Geometry check sheet. Reference: the model listing, model coordinates, mm. A direction names the side the tool comes from. Round coordinates to 2 decimals unless told otherwise and drop trailing zeros. Write each loop counter-clockwise with the first axis right and the second up, starting at its lowest first coordinate (ties: lowest second). Pieces come first, ordered by that corner, then holes. Notation, with made-up numbers: (50.5, 39.5) - (75.5, 39.5) arc R13 ccw to (75.5, 62.5) - close; hole circle Ø10 at (36.5, 4.25). An arc over 180 degrees is marked (long way). Return JSON: item names as keys, results as strings.
```python
from build123d import *

# Parameters (mm, degrees)
ESQUISSE1_W        = 65
ESQUISSE1_H        = 10
BOSS_EXTRU_1_DEPTH = 4
CONG_1_R           = 2
ESQUISSE3_W        = 2.5
ESQUISSE3_H        = 6
BOSS_EXTRU_2_DEPTH = 13
ESQUISSE4_W        = 7
ESQUISSE4_H        = 6
ESQUISSE4_R        = 1.65
BOSS_EXTRU_3_DEPTH = 2


with BuildPart() as part:
    # Esquisse1 → Boss.-Extru.1 (new body)
    with BuildSketch(Plane.XY):
        with Locations((-5.559006211, 7.158385093)):
            Rectangle(ESQUISSE1_W, ESQUISSE1_H)
    extrude(amount=BOSS_EXTRU_1_DEPTH)

    # Congé1
    cong_1_edges = [part.edges().sort_by_distance(p)[0] for p in [
        (-5.559006211, 12.158385093, 4),
        (-5.559006211, 12.158385093, 0),
        (-5.559006211, 2.158385093, 0),
        (-38.059006211, 12.158385093, 2),
        (26.940993789, 12.158385093, 2),
        (26.940993789, 2.158385093, 2),
        (-38.059006211, 2.158385093, 2),
        (-5.559006211, 2.158385093, 4),
    ]]
    fillet(cong_1_edges, radius=CONG_1_R - 0.0001)  # a hair under: the kernel refuses the full size

    # Esquisse3 → Boss.-Extru.2 (add)
    with BuildSketch(Plane.XY.offset(4)):
        with Locations((-36.809006211, 7.158385093)):
            Rectangle(ESQUISSE3_W, ESQUISSE3_H)
        with Locations((25.690993789, 7.158385093)):
            Rectangle(ESQUISSE3_W, ESQUISSE3_H)
    extrude(amount=BOSS_EXTRU_2_DEPTH)

    # Esquisse4 → Boss.-Extru.3 (add)
    with BuildSketch(Plane.XY.offset(17)):
        with Locations((-41.559006211, 7.158385093)):
            Rectangle(ESQUISSE4_W, ESQUISSE4_H)
        with Locations((-41.482556552, 7.092856814)):
            Circle(ESQUISSE4_R, mode=Mode.SUBTRACT)
    extrude(amount=-BOSS_EXTRU_3_DEPTH)


solid = part.part
```
(1) Release check for a two-part mould opening along X. For faces 1 (the face through (-35.559, 7, 10)), 2 (the face through (-5.1, 2.73, 0.6)), 3 (the face through (-37.7, 11.3, 2)) record: pulls with the +X half, pulls with the -X half, needs draft (parallel to the pull), parting line crosses it, or undercut.
Response values:
{"face 1": "undercut", "face 2": "needs draft", "face 3": "pulls with the -X half"}
(2) Section check A-A, the plane z = 10.5. Enter the section's corners in (x, y).
Response values:
{"outline": "(-38.06, 4.16) - (-35.56, 4.16) - (-35.56, 10.16) - (-38.06, 10.16) - close; (24.44, 4.16) - (26.94, 4.16) - (26.94, 10.16) - (24.44, 10.16) - close"}
(3) Access from +Z, -Z, +X, -X, +Y, -Y to the whole of each face (thin tool, end or side, straight path). Record for faces 4 (the face through (-6, 7, 4)), 5 (the face through (-37.9, 10.158, 12)), 6 (the face through (26, 4.158, 10)), 7 (the face through (-38.059, 7, 7)).
Response values:
{"face 4": "+Z, +Y, -Y", "face 5": "+Z, +X, -X, +Y", "face 6": "+Z, +X, -X, -Y", "face 7": "-Z, -X, +Y, -Y"}
(4) Section check D-D, the plane z = 1. Enter the section's corners in (x, y), plus the area to 3 significant figures.
Response values:
{"outline": "(-38.06, 4.16) arc R2 ccw to (-37.06, 2.43) - (25.94, 2.43) arc R2 ccw to (26.94, 4.16) - (26.94, 10.16) arc R2 ccw to (25.94, 11.89) - (-37.06, 11.89) arc R2 ccw to (-38.06, 10.16) - close", "area": "613 mm^2"}
(5) Material ranges on line 1 along X through (y, z) = (7, 15.25); line 2 along X through (y, z) = (5.75, 14.75); line 3 along X through (y, z) = (5, 15.5), recorded low to high. Write a range as [from, to].
Response values:
{"line 1": "x = [-45.06, -43.13], [-39.84, -35.56], [24.44, 26.94]", "line 2": "x = [-38.06, -35.56], [24.44, 26.94]", "line 3": "x = [-45.06, -35.56], [24.44, 26.94]"}
(6) Section check B-B, the plane y = 9.5. Enter the section's corners in (x, z), plus the area to 3 significant figures.
Response values:
{"outline": "(-45.06, 15) - (-38.06, 15) - (-38.06, 0) - (26.94, 0) - (26.94, 17) - (24.44, 17) - (24.44, 4) - (-35.56, 4) - (-35.56, 17) - (-45.06, 17) - close", "area": "339 mm^2"}
(7) Gauge pin test, flat ends, axial feed: pin 1 (3 mm diameter, centred on x = 17.5, y = 7.5, fed in from +Z); pin 2 (7.5 mm diameter, centred on x = -38.5, z = 10.5, fed in from +Y); pin 3 (6 mm diameter, centred on x = -14.5, z = 9, fed in from +Y); pin 4 (3 mm diameter, centred on y = 8.5, z = 4.5, fed in from -X). Record the tip position at first contact, or that the pin passes through.
Response values:
{"pin 1": "stops at z = 4", "pin 2": "stops at y = 10.16", "pin 3": "passes through", "pin 4": "stops at x = -38.06"}
